Check sheet for the modelled part. Datum: model origin and axes. Units: mm. Give positions to 0.01 mm unless a question says otherwise; leave off trailing zeros. Write each loop counter-clockwise with the first axis right and the second up, starting at its lowest first coordinate (ties: lowest second). Pieces come first, ordered by that corner, then holes. Notation, with made-up numbers: (-36, -27) -> (11, -27) arc R13 ccw to (11, -11) -> close; hole circle Ø8 at (82.5, 23.25). An arc over 180 degrees is marked (long way). Answer as a JSON object with one key per item and string values.
from build123d import *

# Parameters (mm, degrees)
F1_DEPTH = 10
F2_SIZE  = 4.99999


# Not quite as in the source:
# - a fillet or chamfer is up to 0.001 mm smaller than in the source, because OpenCascade refuses the exact size


with BuildPart() as f1:
    # F0 (on Top) → F1 (new body)
    with BuildSketch(Plane.XY):
        Polygon((-26.4395750973, 41.8424181081), (-40.7729081464, 36.8424181081), (-51.4395743695, -23.1575818919), align=None)
    extrude(amount=F1_DEPTH)

    # F2 (size 5 in the source; OpenCascade refuses exactly that, so slightly less here)
    f2_edges = [f1.edges().sort_by_distance(p)[0] for p in [
        (-46.106241, 6.842418, 10),
        (-38.939575, 9.342418, 10),
        (-46.106241, 6.842418, 0),
        (-38.939575, 9.342418, 0),
    ]]
    chamfer(f2_edges, length=F2_SIZE)


solid = f1.part
1. Go/stop test with flat-tipped pins: P1, Ø12, axis at x = -30, y = 4.5, coming from the +Z side; P2, Ø5, axis at y = 29.5, z = 3.5, coming from the +X side. Record where each tip stops, or that it passes through.
Determined:
{"P1": "through", "P2": "x = -30.42"}
2. Sectioned sample at C-C, the plane z = 8.25. Enter the section's corners in (x, y).
Determined:
{"outline": "(-42.31, 9.64) -> (-30.46, 40.44) -> (-37.25, 38.07) -> close"}
3. Scan lines: L1, parallel to X at y = 4.5, z = 5.5; L2, parallel to X at y = 14.5, z = 7.5; L3, parallel to Z at x = -40, y = 22. Record each from-to range of solid material in increasing order. Write a range as [from, to].
Determined:
{"L1": "[-46.01, -41.34]", "L2": "[-42.21, -39.63]", "L3": "[1.64, 8.36]"}
4. Sectioned sample at D-D, the plane z = 1.25. Enter the section's corners in (x, y), plus the area to 3 significant figures.
Determined:
{"outline": "(-40.9, 14.68) -> (-31.08, 40.22) -> (-36.71, 38.26) -> close", "area": "62.3 mm^2"}
